For this review, use the dimensioned drawing (mm, ordinates from the lowest corner) and the shaded views. Coordinates: 2 decimals unless noted, no trailing zeros. Write each loop counter-clockwise with the first axis right and the second up, starting at its lowest first coordinate (ties: lowest second). Pieces come first, ordered by that corner, then holes. Notation, with made-up numbers: M 36,-37 L 82,-37 A14 ccw 82,-21 Z; hole C 34,29.5 d9. An arc over 180 degrees is marked long. Return JSON: item names as keys, results as strings.
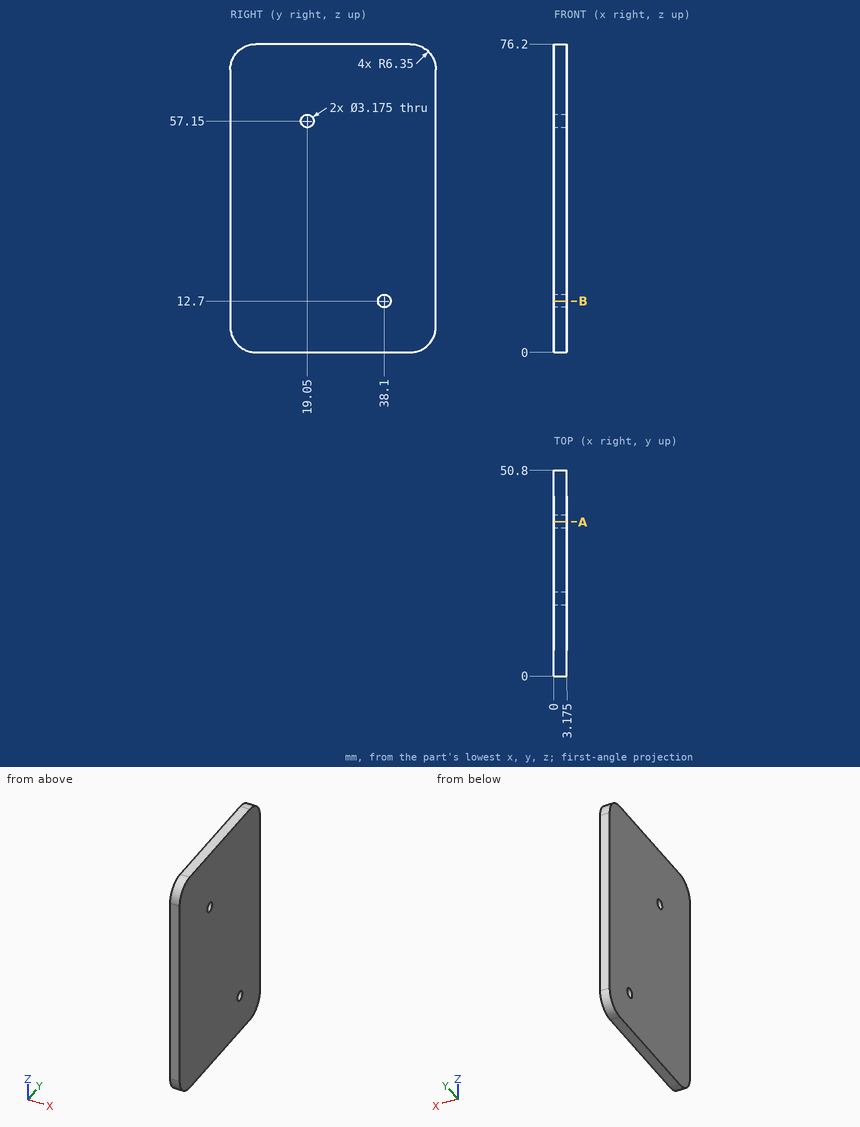
1. Wall thickness on L1, parallel to Z at x = 1.4, y = 19.05; L2, parallel to Z at x = 1.9, y = 38.1; L3, parallel to Y at x = 1.35, z = 12.7: over which ranges is each line inside the solid? List them lowest first. Write a range as from..to.
Checks:
{"L1": "0..55.56, 58.74..76.2", "L2": "0..11.11, 14.29..76.2", "L3": "0..36.51, 39.69..50.8"}
2. We need section A-A (y = 38.1). State the section outline as (x, z) points (1 decimal).
Checks:
{"outline": "M 0,0 L 3.2,0 L 3.2,11.1 L 0,11.1 Z; M 0,14.3 L 3.2,14.3 L 3.2,76.2 L 0,76.2 Z"}
3. We need section B-B (z = 12.7). State the section outline as (x, y) points (1 decimal), plus the area to 3 significant figures.
Checks:
{"outline": "M 0,0 L 3.2,0 L 3.2,36.5 L 0,36.5 Z; M 0,39.7 L 3.2,39.7 L 3.2,50.8 L 0,50.8 Z", "area": "151 mm2"}
